```python
from build123d import *

# Parameters (mm, degrees)
F0_R     = 76.2
F1_DEPTH = 152.4
F2_R     = 25.4
F3_R     = 3.175
F4_DEPTH = 254


with BuildPart() as f1:
    # F0 (on Top) → F1 (new body)
    with BuildSketch(Plane.XY):
        Circle(F0_R)
    extrude(amount=F1_DEPTH)

    # F2
    f2_edges = [f1.edges().sort_by_distance(p)[0] for p in [
        (76.2, 0, 76.2),
        (-76.2, 0, 0),
        (-76.2, 0, 152.4),
    ]]
    fillet(f2_edges, radius=F2_R)

    # F3 (on face) → F4 (cut)
    with BuildSketch(Plane.XY.offset(152.4)):
        Circle(F3_R)
    extrude(amount=-F4_DEPTH, mode=Mode.SUBTRACT)


solid = f1.part
```
Geometry check sheet. Reference: the model listing, model coordinates, mm. Round coordinates to 2 decimals unless told otherwise and drop trailing zeros. Write each loop counter-clockwise with the first axis right and the second up, starting at its lowest first coordinate (ties: lowest second). Pieces come first, ordered by that corner, then holes. Notation, with made-up numbers: (39, 4.25) -> (45, 4.25) arc R25 ccw to (45, 17.25) -> close; hole circle Ø1 at (-6, -33). An arc over 180 degrees is marked (long way). Put each result on its own line as item: value.
1) Cross-section at C-C, the plane z = 123. Enter the section's corners in (x, y) (3 decimals), plus the area to 3 significant figures.
Recorded:
outline: circle Ø152.4 at (0, 0); hole circle Ø6.35 at (0, 0)
area: 18,200 mm2
2) Depth check by flat-ended pin: P1, Ø1.5, axis at y = 13.5, z = 99, coming from the -X side; P2, Ø5, axis at y = -14.5, z = 89.5, coming from the -X side; P3, Ø8, axis at x = 34, z = 130.5, coming from the +Y side. Enter the tip coordinate at first touch or a pass-through.
Recorded:
P1: stops at x = -75.13
P2: stops at x = -75.25
P3: stops at y = 69.86
3) Cross-section at D-D, the plane z = 19.5. Enter the section's corners in (x, y) (3 decimals), plus the area to 3 significant figures.
Recorded:
outline: circle Ø151.011 at (0, 0); hole circle Ø6.35 at (0, 0)
area: 17,900 mm2
4) Cross-section at A-A, the plane x = 0. Enter the section's corners in (y, z) (3 decimals), plus the area to 3 significant figures.
Recorded:
outline: (-76.2, 25.4) arc R25.4 ccw to (-50.8, 0) -> (-3.175, 0) -> (-3.175, 152.4) -> (-50.8, 152.4) arc R25.4 ccw to (-76.2, 127) -> close; (3.175, 0) -> (50.8, 0) arc R25.4 ccw to (76.2, 25.4) -> (76.2, 127) arc R25.4 ccw to (50.8, 152.4) -> (3.175, 152.4) -> close
area: 21,700 mm2
5) Release check for a two-part mould opening along Y. For faces 1 (the face through (-0.69, -3.1, 77.27)), 2 (the face through (11, 1, 152.4)), 3 (the face through (-60.47, -46.367, 75.489)) record: pulls with the +Y half, pulls with the -Y half, needs draft (parallel to the pull), parting line crosses it, or undercut.
Recorded:
face 1: undercut
face 2: needs draft
face 3: parting line crosses it
6) Thickness scan on probe 1 along Y at (x, z) = (0, 43) (3 decimals); probe 2 along X at (y, z) = (-15.5, 84.5); probe 3 along X at (y, z) = (-44.5, 22). Record the ranges inside material, lowest first. Write a range as from..to.
Recorded:
probe 1: y = -76.2..-3.175, 3.175..76.2
probe 2: x = -74.61..74.61
probe 3: x = -61.57..61.57
